The figure shows three views and two pictorial views of one solid part (mm, origin at its lowest corner). Answer the questions. Coordinates: 2 decimals unless noted, no trailing zeros. Order: outer loops, then holes, each group sorted by start corner. A loop starts at its lowest first (then second) coordinate and runs counter-clockwise, first axis right, second up. Notation, with made-up numbers: (71.5, -11) -> (99.5, -11) arc R27 cw to (99.5, 24) -> close; hole circle Ø2 at (41.25, -16). An arc over 180 degrees is marked (long way). Return JSON: item names as keys, results as strings.
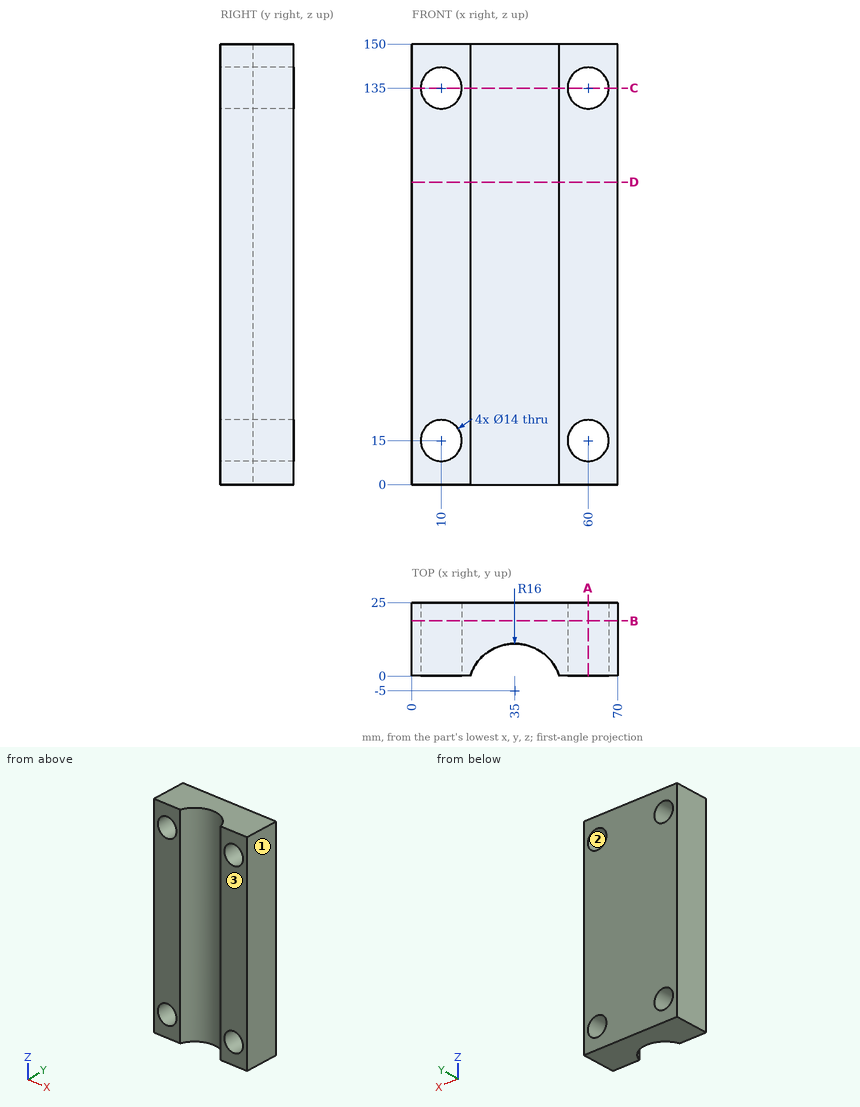
Item 1: The part is cut by section A-A on x = 60. Determine the outline of the cut face in (y, z), plus the area to 3 significant figures.
Answer list:
{"outline": "(0, 0) -> (25, 0) -> (25, 8) -> (0, 8) -> close; (0, 22) -> (25, 22) -> (25, 128) -> (0, 128) -> close; (0, 142) -> (25, 142) -> (25, 150) -> (0, 150) -> close", "area": "3,050 mm2"}
Item 2: Find the intervals of material crossed by probe 1 along Z at (x, y) = (60, 9.5); probe 2 along X at (y, z) = (8.75, 135); probe 3 along X at (y, z) = (6.25, 135), in increasing order.
Answer list:
{"probe 1": "0 to 8, 22 to 128, 142 to 150", "probe 2": "0 to 3, 17 to 26.82, 43.18 to 53, 67 to 70", "probe 3": "0 to 3, 17 to 23.62, 46.38 to 53, 67 to 70"}
Item 3: Determine the mould class of the marked faces 1, 2 and 3 for opening direction X: pulls with the +X half, pulls with the -X half, needs draft (parallel to the pull), parting line crosses it, or undercut.
Answer list:
{"face 1": "pulls with the +X half", "face 2": "undercut", "face 3": "needs draft"}
Item 4: Flat-ended cylindrical pins translate along their axes: pin 1 (10 mm diameter, centred on x = 33, z = 132, fed in from -Y); pin 2 (8.5 mm diameter, centred on x = 10, z = 135, fed in from -Y). Find the tip coordinate at first contact, or state that the pin passes through.
Answer list:
{"pin 1": "y = 9.39", "pin 2": "through"}
Item 5: The part is cut by section C-C on z = 135. Determine the outline of the cut face in (x, y).
Answer list:
{"outline": "(0, 0) -> (3, 0) -> (3, 25) -> (0, 25) -> close; (17, 0) -> (19.8, 0) arc R16 cw to (50.2, 0) -> (53, 0) -> (53, 25) -> (17, 25) -> close; (67, 0) -> (70, 0) -> (70, 25) -> (67, 25) -> close"}
Item 6: The part is cut by section D-D on z = 103. Determine the outline of the cut face in (x, y).
Answer list:
{"outline": "(0, 0) -> (19.8, 0) arc R16 cw to (50.2, 0) -> (70, 0) -> (70, 25) -> (0, 25) -> close"}
Item 7: The part is cut by section B-B on y = 18.75. Determine the outline of the cut face in (x, z), plus the area to 3 significant figures.
Answer list:
{"outline": "(0, 0) -> (70, 0) -> (70, 150) -> (0, 150) -> close; hole circle Ø14 at (10, 15); hole circle Ø14 at (10, 135); hole circle Ø14 at (60, 15); hole circle Ø14 at (60, 135)", "area": "9,880 mm2"}
